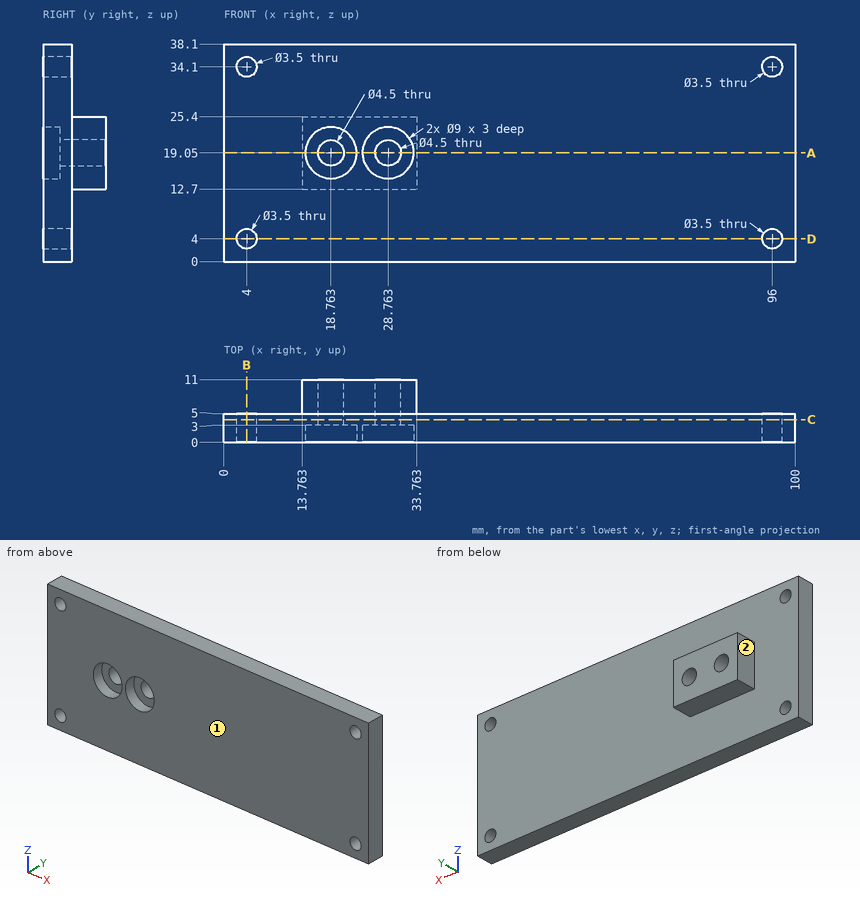
Geometry: see drawing. Coordinates: mm, zero at the bounding-box minimum. A direction names the side the tool comes from. Coordinates: 2 decimals unless noted, no trailing zeros. Order: outer loops, then holes, each group sorted by start corner. A loop starts at its lowest first (then second) coordinate and runs counter-clockwise, first axis right, second up. Notation, with made-up numbers: M -4.75,68.5 L 44.25,68.5 A19 cw 44.25,89.5 Z; hole C 36.5,35 d6. An arc over 180 degrees is marked long. Write each question's results on one line, items separated by ' | '. Start each with the question number.
1) Section query C-C (y = 4). Return the cut outline in (x, z), plus the area to 3 significant figures.
2) Section query A-A (z = 19.05). Return the cut outline in (x, y), plus the area to 3 significant figures.
3) Contact query for flat-ended pins moving along their axis: pin 1 Ø4.5 at (x, z) = (96, 4) entering from +Y; pin 2 Ø4 at (x, z) = (96, 34.1) entering from -Y; pin 3 Ø5 at (x, y) = (19.5, 9.5) entering from +Z; pin 4 Ø5 at (y, z) = (9, 22) entering from -X. Output: stop coordinate, or through.
4) Section query D-D (z = 4). Return the cut outline in (x, y).
5) Line query: line 1 (Z direction, x = 96, y = 2.3); line 2 (X direction, y = 10.5, z = 17) (1 decimal); line 3 (Z direction, x = 29, y = 0.75). Output: solid intervals per line, ascending. Write a range as from..to.
6) Access query for the marked faces 1 and 2. Directions: +Z, -Z, +X, -X, +Y, -Y. A direction counts if a zero-diameter tool reaches every point of the face in a straight line with its end or side. Return the directions, or none.
7) Section query B-B (x = 4). Return the cut outline in (y, z).
Answers:
1) outline: M 0,0 L 100,0 L 100,38.1 L 0,38.1 Z; hole C 4,4 d3.5; hole C 4,34.1 d3.5; hole C 18.76,19.05 d4.5; hole C 28.76,19.05 d4.5; hole C 96,4 d3.5; hole C 96,34.1 d3.5 | area: 3,740 mm^2
2) outline: M 0,0 L 14.26,0 L 14.26,3 L 16.51,3 L 16.51,11 L 13.76,11 L 13.76,5 L 0,5 Z; M 21.01,3 L 23.26,3 L 23.26,0 L 24.26,0 L 24.26,3 L 26.51,3 L 26.51,11 L 21.01,11 Z; M 31.01,3 L 33.26,3 L 33.26,0 L 100,0 L 100,5 L 33.76,5 L 33.76,11 L 31.01,11 Z | area: 494 mm^2
3) pin 1: stops at y = 5 | pin 2: stops at y = 0 | pin 3: stops at z = 25.4 | pin 4: stops at x = 13.76
4) outline: M 0,0 L 2.25,0 L 2.25,5 L 0,5 Z; M 5.75,0 L 94.25,0 L 94.25,5 L 5.75,5 Z; M 97.75,0 L 100,0 L 100,5 L 97.75,5 Z
5) line 1: z = 0..2.25, 5.75..32.35, 35.85..38.1 | line 2: x = 13.8..17.8, 19.7..27.8, 29.7..33.8 | line 3: z = 0..14.56, 23.54..38.1
6) face 1: +Z, -Z, +X, -X, -Y | face 2: +Z, -Z, -X, +Y
7) outline: M 0,0 L 5,0 L 5,2.25 L 0,2.25 Z; M 0,5.75 L 5,5.75 L 5,32.35 L 0,32.35 Z; M 0,35.85 L 5,35.85 L 5,38.1 L 0,38.1 Z
